Geometry: final body of the model. Coordinates: model frame, mm. Coordinates: 2 decimals unless noted, no trailing zeros. Loops run counter-clockwise (first coordinate to the right, second up) from the corner with the lowest first, then second, coordinate; pieces in that order, holes last. Notation, with made-up numbers: M 22,-26.75 L 52,-26.75 A28 cw 52,7.25 Z; hole C 63.5,47 d9. An arc over 180 degrees is marked long. Write each question's results on one line, items separated by ' | '. Start each with the question number.
Autodesk Inventor part; units mm, degrees
ref_plane "YZ Plane" through (0, 0, 0) normal (1, 0, 0) x (0, 1, 0)
ref_plane "XZ Plane" through (0, 0, 0) normal (0, 1, 0) x (-1, 0, 0)
ref_plane "XY Plane" through (0, 0, 0) normal (0, 0, 1) x (1, 0, 0)
sketch "Sketch1" plane through (0, 0, 0) normal (0, 1, 0) x (-1, 0, 0)
  line L0 (-32.5, -55) -> (32.5, -55)
  line L1 (32.5, -55) -> (32.5, 55)
  line L2 (32.5, 55) -> (-32.5, 55)
  line L3 (-32.5, 55) -> (-32.5, -55)
  line L4 (-32.5, -55) -> (32.5, 55) construction
  line L5 (32.5, -55) -> (-32.5, 55) construction
  point P0 (0, 0)
  dimension "Sliding_Plate_Length" = 65
  dimension "Sliding_Plate_Width" = 110
extrude "Extrusion1" add sketch "Sketch1" along normal blind 3
sketch "Sketch2" plane through (0, 3, 0) normal (0, 1, 0) x (1, 0, 0)
  line L0 (-32.5, 55) -> (-32.5, -55)
  line L1 (-32.5, -55) -> (32.5, -55)
  line L2 (32.5, -55) -> (32.5, 55)
  line L3 (32.5, 55) -> (-32.5, 55)
  point P0 (0, 0)
sketch "Sketch3" plane through (0, 3, 0) normal (0, 1, 0) x (1, 0, 0)
  line L0 (15, -50.862) -> (-15, -50.862)
  line L1 (-15, -50.862) -> (-15, -40.862)
  line L2 (-15, -40.862) -> (15, -40.862)
  line L3 (15, -40.862) -> (15, -50.862)
  line L4 (15, -50.862) -> (-15, -40.862) construction
  line L5 (-15, -50.862) -> (15, -40.862) construction
  point P0 (0, 0)
  point P1 (0, -45.862)
  dimension "d6" = 30
  dimension "d7" = 10
extrude "Extrusion2" cut sketch "Sketch3" against normal blind 1.55
properties part number "Rear_Port_Slider"
Item 1: Ray query, L1, parallel to Z at x = 0, y = 2.5; L2, parallel to Y at x = 4.5, z = 42. Return the intervals inside material, ascending. Write a range as [from, to].
Item 2: Pull-direction query (Z, two-part tool) for faces 1 (the flat face through (0, 1, 55)), 2 (the flat face through (0, 0, 1)), 3 (the flat face through (0, 1.45, 46)); classes: released by +Z, released by -Z, zero draft, split by the parting line, or undercut.
Item 3: Contact query for a flat-ended pin moving along its axis: P1, Ø5, axis at x = 4, z = 45, coming from the +Y side. Output: stop coordinate, or through.
Item 4: Section B-B, the plane x = 3.5. Return loops of the section in (y, z).
Item 5: Section A-A, the plane y = 2.55. Return loops of the section in (x, z), plus the area to 3 significant figures.
Solutions:
1) L1: z = [-55, 40.86], [50.86, 55] | L2: y = [0, 1.45]
2) face 1: released by +Z | face 2: zero draft | face 3: undercut
3) P1: stops at y = 1.45
4) outline: M 0,-55 L 3,-55 L 3,40.86 L 1.45,40.86 L 1.45,50.86 L 3,50.86 L 3,55 L 0,55 Z
5) outline: M -32.5,-55 L 32.5,-55 L 32.5,55 L -32.5,55 Z; hole M -15,40.86 L 15,40.86 L 15,50.86 L -15,50.86 Z | area: 6,850 mm²
